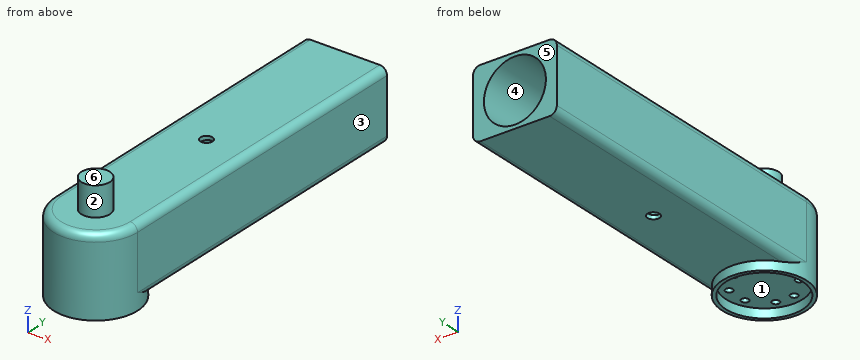
Autodesk Inventor part; units mm, degrees
ref_plane "YZ Plane" through (0, 0, 0) normal (1, 0, 0) x (0, 1, 0)
ref_plane "XZ Plane" through (0, 0, 0) normal (0, 1, 0) x (-1, 0, 0)
ref_plane "XY Plane" through (0, 0, 0) normal (0, 0, 1) x (1, 0, 0)
sketch "Sketch1" plane through (0, 0, 0) normal (0, 0, 1) x (1, 0, 0)
  circle A0 centre (0, 0) radius 11.5
  dimension "d0" = 23
extrude "Extrusion1" add sketch "Sketch1" along normal blind 26
sketch "Sketch2" plane through (0, 0, 0) normal (0, 1, 0) x (-1, 0, 0)
  line L0 (11.5, 0) -> (11.5, 26)
  line L1 (11.5, 26) -> (-11.5, 26)
  line L2 (11.5, 0) -> (-11.5, 0)
  line L3 (-11.5, 0) -> (-11.5, 26)
  line L4 (11.5, 0) -> (-11.5, 19) construction
  line L5 (-11.5, 0) -> (-11.5, 26) construction
  line L6 (-11.5, 0) -> (11.5, 19) construction
  line L7 (11.5, 0) -> (11.5, 26) construction
  line L8 (11.5, 19) -> (-11.5, 19) construction
  line L9 (11.5, 19) -> (-11.5, 19)
  line L10 (-11.5, 19) -> (-11.5, 0)
  line L11 (-11.5, 0) -> (11.5, 0)
  line L12 (11.5, 0) -> (11.5, 19)
  line L13 (11.5, 19) -> (-11.5, 0) construction
  line L14 (-11.5, 19) -> (11.5, 0) construction
  point P0 (0, 0)
  point P1 (11.5, 13)
  point P2 (0, 26)
  point P3 (0, 9.5)
  point P4 (0, 9.5)
  dimension "d15" = 7
extrude "Extrusion2" add sketch "Sketch2" along normal blind 90 contours L2 L3 L9 L0
sketch "Sketch3" plane through (0, 90, 7.5) normal (0, 1, 0) x (1, 0, 0)
  line L0 (-11.5, -11.5) -> (11.5, -11.5) construction
  line L1 (11.5, 7.5) -> (-11.5, 7.5)
  line L2 (11.5, -11.5) -> (11.5, 7.5) construction
  line L3 (-11.5, 7.5) -> (-11.5, -11.5) construction
  line L4 (-11.5, 7.5) -> (11.5, 7.5) construction
  circle A0 centre (0, -2) radius 8.5
  line L5 (11.5, -2) -> (-11.5, -2) construction
  line L6 (0, 7.5) -> (0, -11.5) construction
  dimension "d29" = 17
extrude "Extrusion3" cut sketch "Sketch3" against normal blind 80
sketch "Sketch4" plane through (0, 0, 26) normal (0, 0, 1) x (1, 0, 0)
  circle A0 centre (0, 0) radius 3.9
  circle A1 centre (0, 0) radius 11.5
  dimension "d10" = 7.8
  dimension "d11" = 23
extrude "Extrusion4" cut sketch "Sketch4" against normal blind 7
sketch "Sketch5" plane through (0, 0, 26) normal (0, 0, 1) x (1, 0, 0)
  circle A0 centre (0, 0) radius 3.9
  dimension "d18" = 7.8
extrude "Extrusion5" add sketch "Sketch5" along normal blind 1
sketch "Sketch7" plane through (0, 0, 0) normal (0, 0, -1) x (-1, 0, 0)
  circle A0 centre (0, 0) radius 8 construction
  circle A1 centre (-2.6145, 7.5607) radius 1
  circle A2 centre (2.3849, 7.6363) radius 1
  circle A3 centre (7.531, 2.699) radius 1
  circle A4 centre (7.531, -2.699) radius 1
  circle A5 centre (2.3849, -7.6363) radius 1
  circle A6 centre (-2.6145, -7.5607) radius 1
  circle A7 centre (-7.4681, -2.8684) radius 1
  circle A8 centre (-7.4681, 2.8684) radius 1
  dimension "d31" = 16
  dimension "d32" = 15
  dimension "d33" = 15
  dimension "d34" = 5
  dimension "d35" = 5
  dimension "d36" = 2
  dimension "d37" = 2
  dimension "d38" = 2
  dimension "d39" = 2
  dimension "d40" = 2
  dimension "d41" = 2
  dimension "d42" = 2
  dimension "d43" = 2
extrude "Extrusion7" cut sketch "Sketch7" against normal blind 8
sketch "Sketch8" plane through (0, 0, 0) normal (0, 0, -1) x (-1, 0, 0)
  circle A0 centre (0, 0) radius 11.5
  circle A1 centre (0, 0) radius 10.5
  dimension "d46" = 23
  dimension "d47" = 21
extrude "Extrusion8" add sketch "Sketch8" along normal blind 2.5
fillet "Fillet2" radius 2 5 edges at (0, -11.5, 19) (-11.5, 45, 19) (11.5, 45, 19) (11.5, 45, 0) (-11.5, 45, 0)
sketch "Sketch9" plane through (0, 0, 0) normal (0, 0, -1) x (-1, 0, 0)
  circle A0 centre (0, 40) radius 1.65
  line L0 (-9.5, 90) -> (9.5, 90)
  point P0 (0, 0)
  dimension "d51" = 3.3
  dimension "d52" = 50
extrude "Extrusion9" cut sketch "Sketch9" against normal through all
properties part number "stick_mount"
Model file for the job. Use its own axes, mm. Face numbers are marked on the shaded views. A direction names the side the tool comes from. Round coordinates to 2 decimals unless told otherwise and drop trailing zeros. Write each loop counter-clockwise with the first axis right and the second up, starting at its lowest first coordinate (ties: lowest second). Pieces come first, ordered by that corner, then holes. Notation, with made-up numbers: (-6.75, 48.5) - (4.25, 48.5) arc R19 ccw to (4.25, 61.5) - close; hole circle Ø8 at (77, 4). An arc over 180 degrees is marked (long way). Use CSV: the item, a comma, the result in double quotes. Start each with the question number.
Item 1: Band-saw the part on C-C (y = 58). Write the cut outline in (x, z).
Item 2: Pin check, flat tips, straight feed: P1, Ø2.5, axis at x = -2.38, y = 7.64, coming from the +Z side; P2, Ø3, axis at x = 7.47, y = 2.87, coming from the -Z side; P3, Ø1.5, axis at x = -4.5, z = 9, coming from the -Y side. Stop position of each tip, or through.
Item 3: Band-saw the part on B-B (y = 40). Write the cut outline in (x, z), and give its area (3 significant figures).
Item 4: Band-saw the part on D-D (z = 9.5). Write the cut outline in (x, y), and give its area (3 significant figures).
Item 5: Drill centre lines: L1, parallel to Z at x = 0, y = 27.5; L2, parallel to Y at x = 2.5, z = 3.75; L3, parallel to Z at x = -4.5, y = 64.5. Where is each one in solid material? Low to high. Write a range as [from, to].
Item 6: Band-saw the part on A-A (x = 0). Write the cut outline in (y, z).
Item 7: Tool access for the marked faces 1, 2 and 3: list every direction of +Z, -Z, +X, -X, +Y, -Y with a clear straight run to the whole face (end or side of a thin tool).
Item 8: Two-plate mould, pull along Z, no slides. Class the marked faces 4, 5 and 6: released by +Z, released by -Z, zero draft, split by the parting line, or undercut.
Checked values:
1,outline,"(-11.5, 2) arc R2 ccw to (-9.5, 0) - (9.5, 0) arc R2 ccw to (11.5, 2) - (11.5, 17) arc R2 ccw to (9.5, 19) - (-9.5, 19) arc R2 ccw to (-11.5, 17) - close; hole circle Ø17 at (0, 9.5)"
2,P1,"stops at z = 19"
2,P2,"stops at z = 0"
2,P3,"stops at y = -10.87"
3,outline,"(-11.5, 2) arc R2 ccw to (-9.5, 0) - (-1.65, 0) - (-1.65, 1.16) arc R8.5 cw to (-1.65, 17.84) - (-1.65, 19) - (-9.5, 19) arc R2 ccw to (-11.5, 17) - close; (1.65, 0) - (9.5, 0) arc R2 ccw to (11.5, 2) - (11.5, 17) arc R2 ccw to (9.5, 19) - (1.65, 19) - (1.65, 17.84) arc R8.5 cw to (1.65, 1.16) - close"
3,area,"200 mm²"
4,outline,"(-11.5, 0) arc R11.5 ccw to (11.5, 0) - (11.5, 90) - (8.5, 90) - (8.5, 10) - (-8.5, 10) - (-8.5, 90) - (-11.5, 90) - close"
4,area,"918 mm²"
5,L1,"z = [0, 1], [18, 19]"
5,L2,"y = [-11.22, -8.55], [-6.57, 6.57], [8.55, 10]"
5,L3,"z = [0, 2.29], [16.71, 19]"
6,outline,"(-11.5, -2.5) - (-10.5, -2.5) - (-10.5, 0) - (10.5, 0) - (10.5, -2.5) - (11.5, -2.5) - (11.5, 0) - (38.35, 0) - (38.35, 1) - (10, 1) - (10, 18) - (38.35, 18) - (38.35, 19) - (3.9, 19) - (3.9, 27) - (-3.9, 27) - (-3.9, 19) - (-9.5, 19) arc R2 ccw to (-11.5, 17) - close; (41.65, 0) - (90, 0) - (90, 1) - (41.65, 1) - close; (41.65, 18) - (90, 18) - (90, 19) - (41.65, 19) - close"
7,face 1,"-Z"
7,face 2,"+Z"
7,face 3,"+Z, -Z, +X, +Y, -Y"
8,face 4,"undercut"
8,face 5,"zero draft"
8,face 6,"released by +Z"
